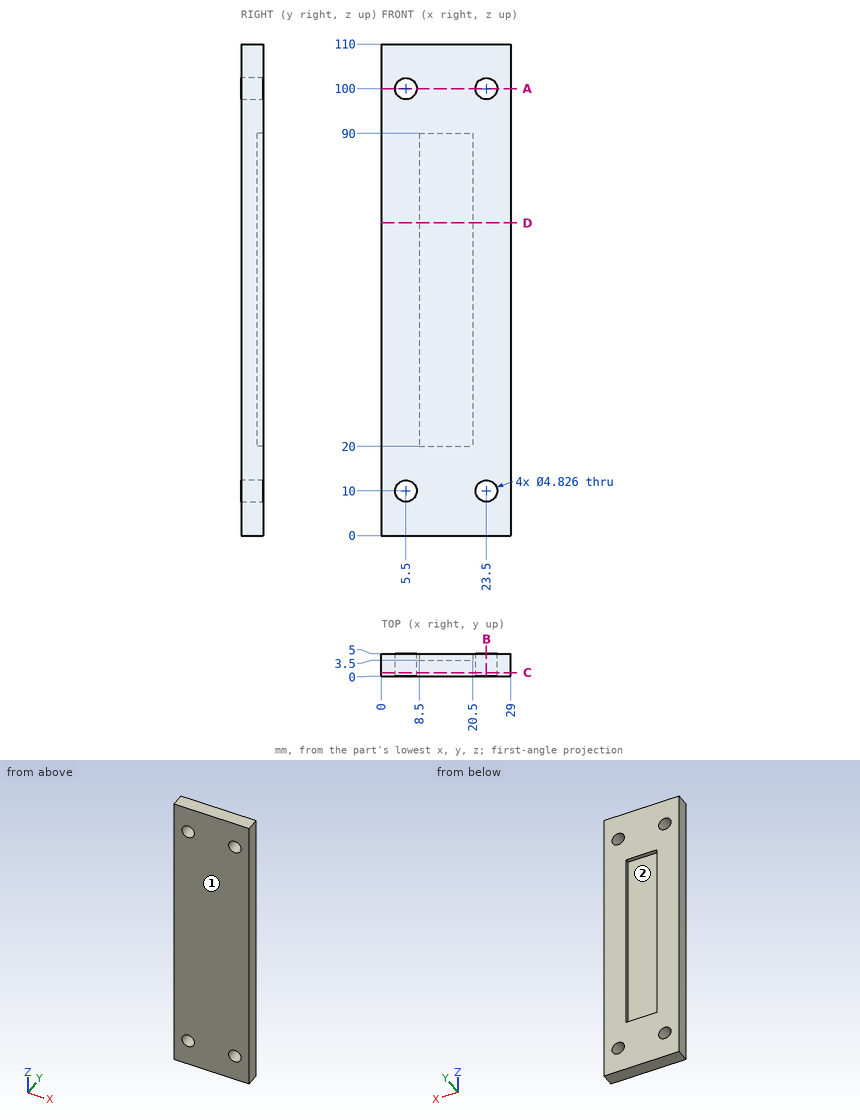
Input: dimensioned drawing with shaded views. Units: mm. Origin: part minimum x, y, z. Round coordinates to 2 decimals unless told otherwise and drop trailing zeros. Loops run counter-clockwise (first coordinate to the right, second up) from the corner with the lowest first, then second, coordinate; pieces in that order, holes last. Notation, with made-up numbers: (25, 83.25) -> (54, 83.25) arc R22 cw to (54, 113.25) -> close; hole circle Ø2 at (69, 31.25). An arc over 180 degrees is marked (long way). Answer as a JSON object with one key per item and string values. Group by question number.
1) Ray query, L1, parallel to X at y = 2.95, z = 100; L2, parallel to X at y = 4.4, z = 65.5; L3, parallel to X at y = 3.7, z = 12. Return the intervals inside material, ascending.
2) Section query D-D on z = 70. Output: boundary loops of the cut face in (x, y).
3) Section query A-A on z = 100. Output: boundary loops of the cut face in (x, y).
4) Draft query along Z for the marked faces 1 and 2. Return one class per face: +Z half, -Z half, draft (parallel to the pull), parting line (faces both ways), or undercut.
5) Section query C-C on y = 0.75. Output: boundary loops of the cut face in (x, z), plus the area to 3 significant figures.
6) Section query B-B on x = 23.5. Output: boundary loops of the cut face in (y, z).
Reply:
{
 "1": {"L1": "x = 0 to 3.09, 7.91 to 21.09, 25.91 to 29", "L2": "x = 0 to 8.5, 20.5 to 29", "L3": "x = 0 to 4.15, 6.85 to 22.15, 24.85 to 29"},
 "2": {"outline": "(0, 0) -> (29, 0) -> (29, 5) -> (20.5, 5) -> (20.5, 3.5) -> (8.5, 3.5) -> (8.5, 5) -> (0, 5) -> close"},
 "3": {"outline": "(0, 0) -> (3.09, 0) -> (3.09, 5) -> (0, 5) -> close; (7.91, 0) -> (21.09, 0) -> (21.09, 5) -> (7.91, 5) -> close; (25.91, 0) -> (29, 0) -> (29, 5) -> (25.91, 5) -> close"},
 "4": {"face 1": "draft", "face 2": "undercut"},
 "5": {"outline": "(0, 0) -> (29, 0) -> (29, 110) -> (0, 110) -> close; hole circle Ø4.83 at (5.5, 10); hole circle Ø4.83 at (5.5, 100); hole circle Ø4.83 at (23.5, 10); hole circle Ø4.83 at (23.5, 100)", "area": "3,120 mm2"},
 "6": {"outline": "(0, 0) -> (5, 0) -> (5, 7.59) -> (0, 7.59) -> close; (0, 12.41) -> (5, 12.41) -> (5, 97.59) -> (0, 97.59) -> close; (0, 102.41) -> (5, 102.41) -> (5, 110) -> (0, 110) -> close"}
}
